The model under review builds one solid part; all positions refer to its coordinate system, in mm. A direction names the side the tool comes from. Coordinates: 2 decimals unless noted, no trailing zeros. Loops run counter-clockwise (first coordinate to the right, second up) from the corner with the lowest first, then second, coordinate; pieces in that order, holes last. Notation, with made-up numbers: M 21,23.25 L 30,23.25 A23 ccw 30,61.25 Z; hole C 4,23 d5. An arc over 180 degrees is marked long. Return JSON: item names as keys, results as strings.
```python
from build123d import *

# Parameters (mm, degrees)
SKETCH1_R           = 45
BOSS_EXTRUDE1_DEPTH = 3


with BuildPart() as part:
    # Sketch1 → Boss-Extrude1 (new body)
    with BuildSketch(Plane(origin=(0, 0, 0), x_dir=(1, 0, 0), z_dir=(0, 1, 0))):
        with Locations(Location((0, 0, 0), (0, 0, 270))):  # turned: the seam where the file's is
            Circle(SKETCH1_R)
        Polygon((18.201594334, 34.879867703), (18.201594334, 27.379867703), (-8.699447333, 27.379867703), (-8.699447333, 8.213201037), (14.881281834, 8.213201037), (14.881281834, 0.713201037), (-8.699447333, 0.713201037), (-8.699447333, -25.120132297), (-17.866113999, -25.120132297), (-17.866113999, 34.879867703), align=None, mode=Mode.SUBTRACT)
    extrude(amount=BOSS_EXTRUDE1_DEPTH)


solid = part.part
```
1. Add section A-A on x = 0. Give the boundary of the cut face in (y, z).
Check values:
{"outline": "M 0,-45 L 3,-45 L 3,-34.88 L 0,-34.88 Z; M 0,-27.38 L 3,-27.38 L 3,-8.21 L 0,-8.21 Z; M 0,-0.71 L 3,-0.71 L 3,45 L 0,45 Z"}
2. Add section C-C on z = -5. Give the boundary of the cut face in (x, y).
Check values:
{"outline": "M -44.72,0 L -17.87,0 L -17.87,3 L -44.72,3 Z; M 14.88,0 L 44.72,0 L 44.72,3 L 14.88,3 Z"}
3. To check wall thickness, follow line 1 (Z direction, x = 4.5, y = 2.85); line 2 (Z direction, x = 5, y = 1.05); line 3 (Z direction, x = -11, y = 2.7). State the ranges of each line that lie inside material, in increasing order.
Check values:
{"line 1": "-44.77 to -34.88, -27.38 to -8.21, -0.71 to 44.77", "line 2": "-44.72 to -34.88, -27.38 to -8.21, -0.71 to 44.72", "line 3": "-43.63 to -34.88, 25.12 to 43.63"}
4. Insertion check: pin 1 Ø0.9 at (y, z) = (1, -30) entering from -X; pin 2 Ø0.9 at (x, y) = (2.5, 1.5) entering from +Z; pin 3 Ø1.5 at (y, z) = (1, 10.5) entering from -X. Each pin has a flat end and moves straight along its axis. Give the tip position at first contact, or say it passes through.
Check values:
{"pin 1": "x = -33.94", "pin 2": "z = 44.95", "pin 3": "x = -43.93"}
5. Add section B-B on x = -16.5. Give the boundary of the cut face in (y, z), plus the area to 3 significant figures.
Check values:
{"outline": "M 0,-41.87 L 3,-41.87 L 3,-34.88 L 0,-34.88 Z; M 0,25.12 L 3,25.12 L 3,41.87 L 0,41.87 Z", "area": "71.2 mm²"}
6. Add section D-D on x = -28. Give the boundary of the cut face in (y, z).
Check values:
{"outline": "M 0,-35.23 L 3,-35.23 L 3,35.23 L 0,35.23 Z"}
7. The part is to be moulded in two halves that separate along X. For faces 3 (the face through (1, 0, 9)), 4 (the face through (-17.235, 1.479, 41.569)), 5 (the face through (18.202, 1, -31)), say which applies: released by +X, released by -X, zero draft, split by the parting line, or undercut.
Check values:
{"face 3": "zero draft", "face 4": "split by the parting line", "face 5": "undercut"}
8. Machinability: for faces 1 (the face through (-13, 1, 25.12)), 2 (the face through (1, 3, 9)), which of the approach directions +Z, -Z, +X, -X, +Y, -Y give a long, thin tool a straight path to every point of the face, cutting with its end or side? Answer none if there is none.
Check values:
{"face 1": "+Y, -Y", "face 2": "+Z, -Z, +X, -X, +Y"}
